Design review of the part built by this model. Coordinates are the model's own, in mm. A direction names the side the tool comes from. Give positions to 0.01 mm unless a question says otherwise; leave off trailing zeros. Write each loop counter-clockwise with the first axis right and the second up, starting at its lowest first coordinate (ties: lowest second). Pieces come first, ordered by that corner, then holes. Notation, with made-up numbers: (11.5, 26.5) -> (43.5, 26.5) arc R22 ccw to (43.5, 60.5) -> close; hole circle Ø1 at (73, 64.5). An arc over 180 degrees is marked (long way). Use CSV: the item, a comma, the result in double quotes.
```python
from build123d import *

# Parameters (mm, degrees)
F1_DEPTH = 6.35
F2_R     = 1.75
F3_DEPTH = 3
F5_DEPTH = 3
F6_R     = 1.75
F7_DEPTH = 3.175
F8_SIZE  = 1.016


with BuildPart() as f1:
    # F0 (on Top) → F1 (new body, symmetric)
    with BuildSketch(Plane.XY):
        with BuildLine():
            Line((40.005, 7.9375), (0, 7.9375))
            Line((0, 7.9375), (0, -7.9375))
            Line((0, -7.9375), (40.005, -7.9375))
            ThreePointArc((40.005, -7.9375), (47.9425, 0), (40.005, 7.9375))
        make_face()
        with BuildLine():
            Line((20.955, -4.7625), (16.51, -4.7625))
            ThreePointArc((16.51, -4.7625), (11.7475, 0), (16.51, 4.7625))
            Line((16.51, 4.7625), (20.955, 4.7625))
            ThreePointArc((20.955, 4.7625), (25.7175, 0), (20.955, -4.7625))
        make_face(mode=Mode.SUBTRACT)
        with BuildLine():
            Line((40.005, -4.7625), (35.56, -4.7625))
            ThreePointArc((35.56, -4.7625), (30.7975, 0), (35.56, 4.7625))
            Line((35.56, 4.7625), (40.005, 4.7625))
            ThreePointArc((40.005, 4.7625), (44.7675, 0), (40.005, -4.7625))
        make_face(mode=Mode.SUBTRACT)
    extrude(amount=F1_DEPTH, both=True)

    # F2 (on face) → F3 (cut)
    with BuildSketch(Plane(origin=(0, 0, 0), x_dir=(0, -1, 0), z_dir=(-1, 0, 0))):
        Circle(F2_R)
    extrude(amount=-F3_DEPTH, mode=Mode.SUBTRACT)

    # F4 (on face) → F5 (cut)
    with BuildSketch(Plane(origin=(3, 0, 0), x_dir=(0, -1, 0), z_dir=(-1, 0, 0))):
        Polygon((2.9845, -1.7231018784), (2.9845, 1.7231018784), (2.9845, 6.35), (-2.9845, 6.35), (-2.9845, 1.7231018784), (-2.9845, -1.7231018784), (0, -3.4462037568), align=None)
    extrude(amount=-F5_DEPTH, mode=Mode.SUBTRACT)

    # F6 (on face) → F7 (cut)
    with BuildSketch(Plane(origin=(6, 0, 0), x_dir=(0, -1, 0), z_dir=(-1, 0, 0))):
        Circle(F6_R)
    extrude(amount=-F7_DEPTH, mode=Mode.SUBTRACT)

    # F8
    f8_edges = [f1.edges().sort_by_distance(p)[0] for p in [
        (20.0025, -7.9375, 6.35),
        (20.0025, -7.9375, -6.35),
        (25.7175, 0, 6.35),
        (30.7975, 0, 6.35),
        (30.7975, 0, -6.35),
        (25.7175, 0, -6.35),
    ]]
    chamfer(f8_edges, length=F8_SIZE)


solid = f1.part
```
(1) Clearance check with a flat-ended pin moving along its axis: pin 1 (1 mm diameter, centred on y = 4.5, z = -2.5, fed in from +X). State where the tip first meets the part, or that it passes through.
Established:
pin 1,"stops at x = 46.86"
(2) Take a section at A-A (x = 19). Write out the cut boundary in (y, z).
Established:
outline,"(-7.94, -5.33) -> (-6.92, -6.35) -> (-5.78, -6.35) -> (-4.76, -5.33) -> (-4.76, 5.33) -> (-5.78, 6.35) -> (-6.92, 6.35) -> (-7.94, 5.33) -> close; (4.76, -5.33) -> (5.78, -6.35) -> (6.92, -6.35) -> (7.94, -5.33) -> (7.94, 5.33) -> (6.92, 6.35) -> (5.78, 6.35) -> (4.76, 5.33) -> close"
(3) Take a section at D-D (z = -2.75). Write out the cut boundary in (x, y) (1 decimal), then the cut area to 3 significant figures.
Established:
outline,"(0, -7.9) -> (40, -7.9) arc R7.9 ccw to (40, 7.9) -> (0, 7.9) -> close; hole (3, -1.2) -> (6, -1.2) -> (6, 1.2) -> (3, 1.2) -> close; hole (16.5, -4.8) -> (21, -4.8) arc R4.8 ccw to (21, 4.8) -> (16.5, 4.8) arc R4.8 ccw to start; hole (35.6, -4.8) -> (40, -4.8) arc R4.8 ccw to (40, 4.8) -> (35.6, 4.8) arc R4.8 ccw to start"
area,"500 mm2"
(4) For line 1 along Z through (x, y) = (2.05, 0); line 2 along X through (y, z) = (-4.25, 3.5); line 3 along X through (y, z) = (-3.5, -2.25), list the stretches that pass through material, from the lowest coordinate up. Write a range as [from, to].
Established:
line 1,"z = [-6.35, -1.75], [1.75, 6.35]"
line 2,"x = [0, 14.36], [23.1, 33.41], [42.15, 46.71]"
line 3,"x = [0, 13.28], [24.18, 32.33], [43.23, 47.13]"
(5) Take a section at B-B (z = 0). State how many separate pieces and enclosed holes the cut face has, then the cut area to 3 significant figures.
Established:
separate pieces,"1"
enclosed holes,"2"
area,"467 mm2"
(6) Take a section at C-C (z = 3). Write out the cut boundary in (x, y) (1 decimal), then the cut area to 3 significant figures.
Established:
outline,"(0, -7.9) -> (40, -7.9) arc R7.9 ccw to (40, 7.9) -> (0, 7.9) -> close; hole (3, -3) -> (6, -3) -> (6, 3) -> (3, 3) -> close; hole (16.5, -4.8) -> (21, -4.8) arc R4.8 ccw to (21, 4.8) -> (16.5, 4.8) arc R4.8 ccw to start; hole (35.6, -4.8) -> (40, -4.8) arc R4.8 ccw to (40, 4.8) -> (35.6, 4.8) arc R4.8 ccw to start"
area,"489 mm2"
(7) Mouldability with a two-part tool opening along Y and no side actions: class faces 6 (the face through (4.479, 1.513, -2.573)), 7 (the face through (0, 2, 0)), 8 (the face through (20.28, 7.44, 5.83)) as +Y half, -Y half, draft (parallel to the pull), parting line (faces both ways), or undercut.
Established:
face 6,"undercut"
face 7,"draft"
face 8,"+Y half"
(8) Tool access review of faces 1 (the face through (18.76, -5.26, 5.83)), 2 (the face through (37.75, 5.26, -5.83)), 3 (the face through (9.175, 0, 0)), 4 (the face through (47.101, -0.156, -6.174)), 5 (the face through (19, -4.762, 0)): name each direction out of +Z, -Z, +X, -X, +Y, -Y from which nothing blocks a thin tool from reaching the whole face with its end or side.
Established:
face 1,"+Z"
face 2,"-Z"
face 3,"-X"
face 4,"-Z, +X"
face 5,"+Z, -Z"
